Build history of the part. All positions in model axes, mm. Give positions to 0.01 mm unless a question says otherwise; leave off trailing zeros. Answer in a Markdown table with one row per item. Add a question column.
from build123d import *

# Parameters (mm, degrees)
F0_R      = 127
F1_DEPTH  = 6.35
F4_DEPTH  = 12.7
F5_R      = 12.5
F6_DEPTH  = 10
F8_SIZE   = 2
F9_W      = 28.838306
F9_H      = 155.121999
F10_DEPTH = 12.7
F11_W     = 82
F11_H     = 6.4
F12_DEPTH = 7
F13_R     = 1


with BuildPart() as f1:
    # F0 (on Top) → F1 (new body, symmetric)
    with BuildSketch(Plane.XY):
        Circle(F0_R)
    extrude(amount=F1_DEPTH, both=True)

    # F3 (on face) → F4 (cut, through all)
    with BuildSketch(Plane.XY.offset(6.35)):
        with BuildLine():
            ThreePointArc((-18.117333, -67.614808), (-70, 0), (-18.117333, 67.614808))
            ThreePointArc((-18.117333, 67.614808), (-3.975198, 92.109705), (-28.470095, 106.251841))
            ThreePointArc((-28.470095, 106.251841), (-110, 0), (-28.470095, -106.251841))
            ThreePointArc((-28.470095, -106.251841), (-3.975198, -92.109705), (-18.117333, -67.614808))
        make_face()
    extrude(amount=-F4_DEPTH, mode=Mode.SUBTRACT)

    # F5 (on face) → F6 (cut)
    with BuildSketch(Plane.XY.offset(6.35)):
        with Locations((-47.631397, 27.5)):
            Circle(F5_R)
        with Locations((-55, 0)):
            Circle(F5_R)
        with Locations((-47.631397, -27.5)):
            Circle(F5_R)
    extrude(amount=-F6_DEPTH, mode=Mode.SUBTRACT)

    # F8
    f8_edges = [f1.edges().sort_by_distance(p)[0] for p in [
        (-110, 0, 6.35),
        (-127, 0, 6.35),
    ]]
    chamfer(f8_edges, length=F8_SIZE)

    # F9 (on face) → F10 (cut, through all)
    with BuildSketch(Plane.XY.offset(6.35)):
        with Locations((124.419153, -2.012827)):
            Rectangle(F9_W, F9_H)
    extrude(amount=-F10_DEPTH, mode=Mode.SUBTRACT)

    # F11 (on face) → F12 (cut)
    with BuildSketch(Plane(origin=(0, 0, -6.35), x_dir=(1, 0, 0), z_dir=(0, 0, -1))):
        with Locations((41, 0)):
            Rectangle(F11_W, F11_H)
    extrude(amount=-F12_DEPTH, mode=Mode.SUBTRACT)

    # F13
    f13_edges = [f1.edges().sort_by_distance(p)[0] for p in [
        (0, -3.2, -2.85),
        (0, 3.2, -2.85),
        (82, 3.2, -2.85),
        (82, -3.2, -2.85),
    ]]
    fillet(f13_edges, radius=F13_R)


solid = f1.part
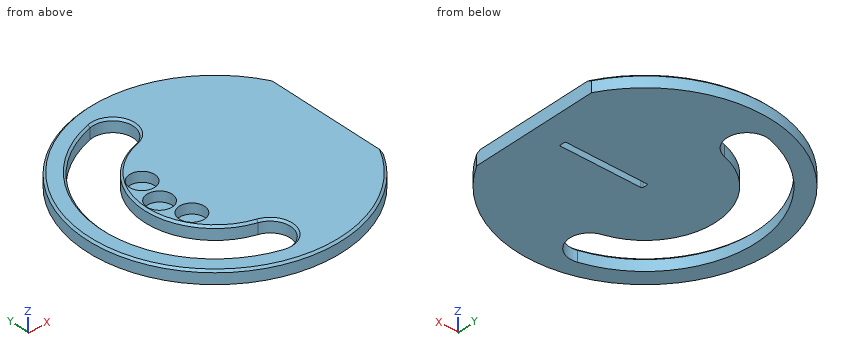
(1) Saw through at A-A, the plane x = -55. State how many separate pieces and enclosed holes the cut face has, then the cut area to 3 significant figures.
(2) Wall check: line 1 along Y through (x, z) = (-41.5, 5); line 2 along X through (y, z) = (-5, 0.5); line 3 along Y through (x, z) = (-10, -0.5). Give the ranges that are in metal, low to high. Write a range as from..to.
(3) Flat gauge pins, fed straight in: pin 1 Ø4 at (x, z) = (35.5, 1) entering from -Y; pin 2 Ø7.5 at (x, y) = (-53.5, 28) entering from +Z; pin 3 Ø3 at (x, z) = (-30, -2.5) entering from +Y; pin 4 Ø7 at (x, y) = (38, -0.5) entering from -Z. Where does each tip first touch, or does it go through?
Worked answers:
| question | item | result |
|---|---|---|
| 1 | separate pieces | 3 |
| 1 | enclosed holes | 0 |
| 1 | area | 918 mm^2 |
| 2 | line 1 | -119.34..-102.57, -55.56..-38.39, -16.61..16.61, 38.39..55.56, 102.57..119.34 |
| 2 | line 2 | -126.9..-109.89, -69.82..-66.46, -43.54..110 |
| 2 | line 3 | -126.61..-101.88, -71.99..71.99, 101.88..126.61 |
| 3 | pin 1 | y = -122.5 |
| 3 | pin 2 | z = -3.65 |
| 3 | pin 3 | y = 123.76 |
| 3 | pin 4 | z = -6.35 |
